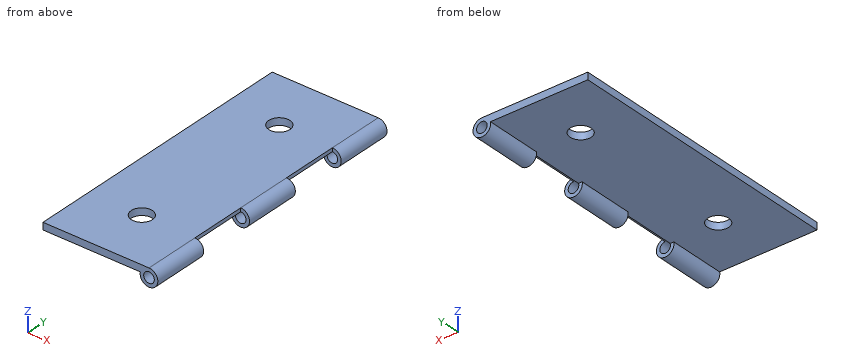
from build123d import *

# Parameters (mm, degrees)
SKETCH1_W           = 15
SKETCH1_H           = 40
SKETCH1_R           = 1.5
BOSS_EXTRUDE2_DEPTH = 1
SKETCH2_R           = 1.25
BOSS_EXTRUDE3_DEPTH = 8
SKETCH3_R           = 0.75
CUT_EXTRUDE1_DEPTH  = 40
LPATTERN1_COUNT     = 3
LPATTERN1_PITCH     = 16
SKETCH4_R           = 0.75
CUT_EXTRUDE2_DEPTH  = 40


with BuildPart() as part:
    # Sketch1 → Boss-Extrude2 (new body)
    with BuildSketch(Plane.XY):
        Rectangle(SKETCH1_W, SKETCH1_H)
        with Locations((0, 12)):
            Circle(SKETCH1_R, mode=Mode.SUBTRACT)
        with Locations((0, -12)):
            Circle(SKETCH1_R, mode=Mode.SUBTRACT)
    extrude(amount=BOSS_EXTRUDE2_DEPTH)

    # Sketch2 → Boss-Extrude3 (add)
    with BuildSketch(Plane(origin=(0, 20, 0), x_dir=(1, 0, 0), z_dir=(0, 1, 0))):
        with Locations((7.5, 0.25)):
            Circle(SKETCH2_R)
    boss_extrude3 = extrude(amount=-BOSS_EXTRUDE3_DEPTH)

    # Sketch3 → Cut-Extrude1 (cut)
    with BuildSketch(Plane(origin=(0, 20, 0), x_dir=(1, 0, 0), z_dir=(0, 1, 0))):
        with Locations((7.5, 0.25)):
            Circle(SKETCH3_R)
    extrude(amount=-CUT_EXTRUDE1_DEPTH, mode=Mode.SUBTRACT)

    # LPattern1: Boss-Extrude3 ×3
    with Locations(*[(0, -i * LPATTERN1_PITCH, 0) for i in range(1, LPATTERN1_COUNT)]):
        add(boss_extrude3)

    # Sketch4 → Cut-Extrude2 (cut)
    with BuildSketch(Plane(origin=(0, 20, 0), x_dir=(1, 0, 0), z_dir=(0, 1, 0))):
        with Locations((7.5, 0.25)):
            Circle(SKETCH4_R)
    extrude(amount=-CUT_EXTRUDE2_DEPTH, mode=Mode.SUBTRACT)


solid = part.part
Check sheet for the modelled part. Datum: model origin and axes. Units: mm. Round coordinates to 2 decimals unless told otherwise and drop trailing zeros. Order: outer loops, then holes, each group sorted by start corner. A loop starts at its lowest first (then second) coordinate and runs counter-clockwise, first axis right, second up.
(1) Cross-section at A-A, the plane x = 0. Enter the section's corners in (y, z).
(2) Cross-section at C-C, the plane x = 3.5. Enter the section's corners in (y, z).
(3) Cross-section at B-B, the plane y = 8.5. Enter the section's corners in (x, z), and give its area (3 significant figures).
(4) Go/stop test with flat-tipped pins: P1, Ø0.8, axis at x = 7, z = 0, coming from the +Y side; P2, Ø4.5, axis at x = -3.5, y = -0.5, coming from the -Z side; P3, Ø0.9, axis at x = 7.5, z = -0.25, coming from the -Y side. Record where each tip stops, or that it passes through.
(5) Scan lines: probe 1 along Y at (x, z) = (0, 0.2); probe 2 along Z at (x, y) = (7.5, 3); probe 3 along X at (y, z) = (3, -0.25). Record each from-to range of solid material in increasing order.
Check sheet entries:
1. outline: (-20, 0) - (-13.5, 0) - (-13.5, 1) - (-20, 1) - close; (-10.5, 0) - (10.5, 0) - (10.5, 1) - (-10.5, 1) - close; (13.5, 0) - (20, 0) - (20, 1) - (13.5, 1) - close
2. outline: (-20, 0) - (20, 0) - (20, 1) - (-20, 1) - close
3. outline: (-7.5, 0) - (6.79, 0) arc R0.75 cw to (7.5, 0.5) - (7.5, 1) - (-7.5, 1) - close
3. area: 14.7 mm2
4. P1: stops at y = 20
4. P2: stops at z = 0
4. P3: passes through
5. probe 1: y = -20 to -13.5, -10.5 to 10.5, 13.5 to 20
5. probe 2: z = -1.5 to -1, 0.5 to 1
5. probe 3: x = 6.25 to 6.75, 8.25 to 8.75
